Geometry: final body of the model. Coordinates: model frame, mm. Face numbers are marked on the shaded views. A direction names the side the tool comes from. Coordinates: 2 decimals unless noted, no trailing zeros. Loops run counter-clockwise (first coordinate to the right, second up) from the corner with the lowest first, then second, coordinate; pieces in that order, holes last. Notation, with made-up numbers: (53, 21.5) - (84, 21.5) arc R22 cw to (84, 45.5) - close; hole circle Ø6 at (-15, 67.25). An arc over 180 degrees is marked (long way). Answer in a Markdown table with one row per item.
from build123d import *

# Parameters (mm, degrees)
SKETCH1_W               = 220
SKETCH1_H               = 120
BOSS_EXTRUDE1_DEPTH     = 20
SKETCH2_W               = 178.8
SKETCH2_H               = 55.1
CUT_EXTRUDE1_DEPTH      = 2.1
SKETCH3_R               = 5
CUT_EXTRUDE2_DEPTH      = 2
CUT_EXTRUDE3_DEPTH      = 127.571758303
CUT_EXTRUDE3_DEPTH_BACK = 127.571758303
SKETCH4_W               = 74
SKETCH4_H               = 57.1


with BuildPart() as part:
    # Sketch1 → Boss-Extrude1 (new body)
    with BuildSketch(Plane(origin=(0, 0, 0), x_dir=(1, 0, 0), z_dir=(0, 1, 0))):
        Rectangle(SKETCH1_W, SKETCH1_H)
    extrude(amount=-BOSS_EXTRUDE1_DEPTH)

    # Sketch2 → Cut-Extrude1 (cut)
    with BuildSketch(Plane(origin=(0, 0, 0), x_dir=(1, 0, 0), z_dir=(0, 1, 0))):
        Rectangle(SKETCH2_W, SKETCH2_H)
    extrude(amount=-CUT_EXTRUDE1_DEPTH, mode=Mode.SUBTRACT)

    # Sketch3 → Cut-Extrude2 (cut)
    with BuildSketch(Plane(origin=(0, 0, 0), x_dir=(1, 0, 0), z_dir=(0, 1, 0))):
        with Locations((-89.4, 27.55)):
            Circle(SKETCH3_R)
        with Locations((89.4, 27.55)):
            Circle(SKETCH3_R)
        with Locations((89.4, -27.55)):
            Circle(SKETCH3_R)
        with Locations((-89.4, -27.55)):
            Circle(SKETCH3_R)
    extrude(amount=-CUT_EXTRUDE2_DEPTH, mode=Mode.SUBTRACT)

    # Sketch4 → Cut-Extrude3 (cut, two sides: drawn at the far end of the back side and taken through both)
    with BuildSketch(Plane(origin=(0, -2.1, 0), x_dir=(1, 0, 0), z_dir=(0, 1, 0)).offset(-CUT_EXTRUDE3_DEPTH_BACK)):
        Rectangle(SKETCH4_W, SKETCH4_H)
    extrude(amount=CUT_EXTRUDE3_DEPTH + CUT_EXTRUDE3_DEPTH_BACK, mode=Mode.SUBTRACT)


solid = part.part
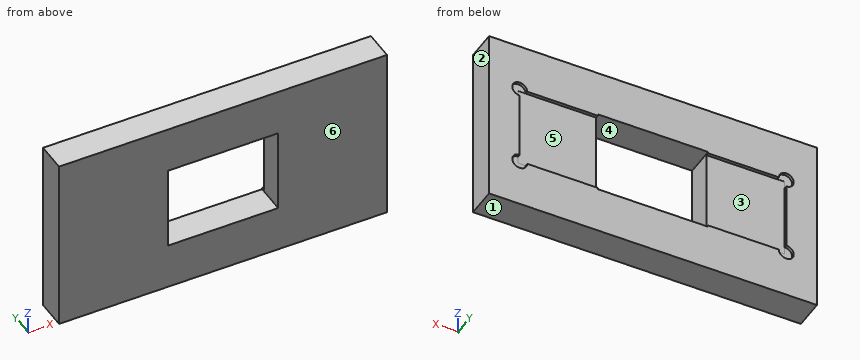
(1) Access query for the marked faces 4, 5 and 6. Directions: +Z, -Z, +X, -X, +Y, -Y. A direction counts if a zero-diameter tool reaches every point of the face in a straight line with its end or side. Return the directions, or none.
Verdict:
| item | result |
|---|---|
| face 4 | +Y, -Y |
| face 5 | +Y |
| face 6 | +Z, -Z, +X, -X, -Y |
(2) Cut plane B-B on y = -9.75. Output: boundary loops of the cut face in (x, z).
Verdict:
| item | result |
|---|---|
| outline | (-110, -60) - (110, -60) - (110, 60) - (-110, 60) - close; hole (-37, -28.55) - (37, -28.55) - (37, 28.55) - (-37, 28.55) - close |
(3) Pull-direction query (X, two-part tool) for the marked faces 1, 2 and 3; classes: pulls with the +X half, pulls with the -X half, needs draft (parallel to the pull), parting line crosses it, or undercut.
Verdict:
| item | result |
|---|---|
| face 1 | needs draft |
| face 2 | pulls with the +X half |
| face 3 | undercut |
(4) Ray query, probe 1 along X at (y, z) = (-5, 14.5); probe 2 along Z at (x, y) = (-4.5, -4.5); probe 3 along Y at (x, z) = (-88.5, -12). Return the intervals inside material, ascending.
Verdict:
| item | result |
|---|---|
| probe 1 | x = -110 to -37, 37 to 110 |
| probe 2 | z = -60 to -28.55, 28.55 to 60 |
| probe 3 | y = -20 to -2.1 |
(5) Cut plane A-A on x = 4. Output: boundary loops of the cut face in (y, z), then the cut area to 3 significant figures.
Verdict:
| item | result |
|---|---|
| outline | (-20, -60) - (0, -60) - (0, -28.55) - (-20, -28.55) - close; (-20, 28.55) - (0, 28.55) - (0, 60) - (-20, 60) - close |
| area | 1,260 mm² |
(6) Cut plane C-C on x = 59.5. Output: boundary loops of the cut face in (y, z).
Verdict:
| item | result |
|---|---|
| outline | (-20, -60) - (0, -60) - (0, -27.55) - (-2.1, -27.55) - (-2.1, 27.55) - (0, 27.55) - (0, 60) - (-20, 60) - close |
(7) First-contact query: pin 1 Ø3 at (x, z) = (-87.5, -27) entering from +Y; pin 2 Ø15.5 at (x, z) = (-56, 7) entering from +Y. Flat tips, straight axial feed; report the tip coordinate or a pass-through.
Verdict:
| item | result |
|---|---|
| pin 1 | stops at y = -2 |
| pin 2 | stops at y = -2.1 |
